```python
from build123d import *

# Parameters (mm, degrees)
F2_SIZE = 1
F3_SIZE = 2
F4_R    = 4


with BuildPart() as f1:
    # F0 (on Front) → F1 (revolve)
    with BuildSketch(Plane.XZ):
        Polygon((0, 23.5), (-5, 23.5), (-5, 20.5), (0, 20.5), (6.887489, 13.25), (26.887489, 13.25), (26.887489, 16.25), (6.887489, 16.25), align=None)
    revolve(axis=Axis((9.662958, 0, 0), (1, 0, 0)))

    # F2
    f2_edges = [f1.edges().sort_by_distance(p)[0] for p in [
        (-5, 0, -23.5),
    ]]
    chamfer(f2_edges, length=F2_SIZE)

    # F3
    f3_edges = [f1.edges().sort_by_distance(p)[0] for p in [
        (26.887489, 0, -16.25),
    ]]
    chamfer(f3_edges, length=F3_SIZE)

    # F4
    f4_edges = [f1.edges().sort_by_distance(p)[0] for p in [
        (6.887489, 0, -16.25),
        (6.887489, 0, -13.25),
        (0, 0, -20.5),
    ]]
    fillet(f4_edges, radius=F4_R)


solid = f1.part
```
The listing builds one solid part. Answer for the finished solid, in the listing's coordinates (mm). A direction names the side the tool comes from. Round coordinates to 2 decimals unless told otherwise and drop trailing zeros. Write each loop counter-clockwise with the first axis right and the second up, starting at its lowest first coordinate (ties: lowest second). Pieces come first, ordered by that corner, then holes. Notation, with made-up numbers: (62, 77) -> (102, 77) arc R26 cw to (102, 92) -> close; hole circle Ø3 at (-25.75, 65.5). An arc over 180 degrees is marked (long way). Answer as a JSON object with one key per item and string values. Group by question number.
Q1. Each of these flat-tipped pins is pushed along its axis until it touches: pin 1 Ø6 at (x, z) = (14, -12.5) entering from -Y; pin 2 Ø6 at (x, z) = (10, 16) entering from -Y; pin 3 Ø8 at (x, y) = (-2, 7) entering from +Z. Where does it stop, or does it pass through?
Q2. Section A-A (x = 20.5) is taken. Write down the section's boundary in (y, z), plus the area to 3 significant figures.
Q3. Which of the six approach directions +Z, -Z, +X, -X, +Y, -Y give full straight-line access (tool end or side, diameter ignored) to faces 1 (the face through (-2, -7.1, 22.4)), 2 (the face through (-3.34, 12.47, -16.27)), 3 (the face through (16.63, -4.88, 15.5))?
Q4. Straight lines are drawn through the part: line 1 along Z through (x, y) = (23, 0); line 2 along Z through (x, y) = (-4, 0). For each, find the intervals that lie inside material, in ascending order.
Check values:
{
 "1": {"pin 1": "y = -13.18", "pin 2": "y = -9.75", "pin 3": "z = 23.31"},
 "2": {"outline": "circle Ø32.5 at (0, 0); hole circle Ø26.5 at (0, 0)", "area": "278 mm^2"},
 "3": {"face 1": "+X, -X", "face 2": "-X", "face 3": "+X"},
 "4": {"line 1": "-16.25 to -13.25, 13.25 to 16.25", "line 2": "-23.5 to -20.5, 20.5 to 23.5"}
}
